Can you work these out from the model? Positions are in its coordinate system, mm. A direction names the side the tool comes from. Give positions to 0.01 mm unless a question says otherwise; leave off trailing zeros. Write each loop counter-clockwise with the first axis right and the second up, starting at its lowest first coordinate (ties: lowest second). Pieces come first, ordered by that corner, then holes. Notation, with made-up numbers: (8.25, 57.25) -> (27.25, 57.25) arc R28 ccw to (27.25, 91.25) -> close; hole circle Ø6 at (-14, 82). An arc over 180 degrees is marked (long way). Answer as CSV lines item,"result". Start each with the question number.
1. I need wall thicknesses on line 1 (X direction, y = -3.5, z = 160); line 2 (Z direction, x = -81.5, y = 8.5); line 3 (X direction, y = 13, z = 170). Which ranges of each line are inside material? Lowest first, please. Write a range as [from, to].
2. If we section it at B-B on y = -6.5: Write out the boundary of the cut face in (x, z).
3. I'm going to push flat-ended pins straight in: P1, Ø5, axis at y = 20, z = 117, coming from the -X side; P2, Ø5, axis at y = 20.5, z = 169.5, coming from the +X side; P3, Ø9.5, axis at y = 10, z = 165.5, coming from the -X side; P4, Ø4, axis at x = -64.5, z = 109, coming from the -Y side. Where does each tip first touch, or does it pass through?
4. If we section it at A-A on z = 135: Write out the boundary of the cut face in (x, y), plus the area to 3 significant figures.
5. If we mould it in two halves opening along X, with no side actions, what happens to faces 1 (the face through (-106.579, 10, 169)), 2 (the face through (-67.574, -4.93, 159.78)), 3 (the face through (-29.5, -4.9, 107.5)), 4 (the face through (-92, -3, 91))? For each: pulls with the +X half, pulls with the -X half, needs draft (parallel to the pull), parting line crosses it, or undercut.
6. If we section it at C-C on x = -109.5: Write out the boundary of the cut face in (y, z), plus the area to 3 significant figures.
7. On a 3-axis mill with a long thin cutter (end or side, diameter ignored), from which of +Z, -Z, +X, -X, +Y, -Y can I reach the whole of each face in a straight line? I mean faces 5 (the face through (-106.579, 10, 100)), 6 (the face through (-93.579, 15, 99)), 7 (the face through (-90.579, 15, 150)). Say none if no direction works.
Autodesk Fusion 360 part; units mm, degrees
sketch "Sketch1" plane through (0, 0, 0) normal (0, 1, 0) x (1, 0, 0)
  line L0 (-93.5789, -91) -> (-48.797, -91)
  line L1 (-48.797, -91) -> (-48.797, -179)
  line L2 (-48.797, -179) -> (-93.5789, -179)
  line L3 (-93.5789, -179) -> (-93.5789, -91)
  line L4 (-48.797, -179) -> (2.6553, -135)
  line L5 (2.6553, -135) -> (-48.797, -91)
  line L6 (-93.5789, -91) -> (-148.2679, -91)
  line L7 (-148.2679, -91) -> (-148.2679, -179)
  line L8 (-148.2679, -179) -> (-93.5789, -179)
  line L9 (2.6553, -135) -> (-148.2679, -135)
  line L10 (-90.5789, -91) -> (-90.5789, -179)
  line L11 (-26.5789, -110) -> (-26.5789, -160)
  line L12 (-26.5789, -130) -> (-90.5789, -130)
  line L13 (-26.5789, -140) -> (-90.5789, -140)
  line L14 (-26.5789, -110) -> (-90.5789, -110)
  line L15 (-26.5789, -160) -> (-90.5789, -160)
  line L16 (-62.5789, -91) -> (-62.5789, -179)
  circle A0 centre (-62.5789, -110) radius 5
  circle A1 centre (-62.5789, -160) radius 5
  line L17 (-106.5789, -91) -> (-106.5789, -179)
  line L18 (-112.5789, -91) -> (-112.5789, -179)
  line L19 (-86.5789, -140) -> (-86.5789, -130)
  circle A2 centre (-112.5789, -135) radius 9.5
  circle A3 centre (-112.5789, -135) radius 19
  line L20 (-26.5789, -135) -> (-14.2304, -120.56)
  line L21 (-26.5789, -135) -> (-14.2304, -149.44)
  circle A4 centre (-26.5789, -135) radius 19
  line L22 (-90.5789, -160) -> (-93.5789, -160)
  line L23 (-90.5789, -130) -> (-93.5789, -130)
  line L24 (-90.5789, -110) -> (-93.5789, -110)
  line L25 (-90.5789, -140) -> (-93.5789, -140)
  dimension "d1" = 3
  dimension "d2" = 5
  dimension "d3" = 10
  dimension "d4" = 50
  dimension "d7" = 88
  dimension "d8" = 67
  dimension "d10" = 31
  dimension "d11" = 36
  dimension "d12" = 10
  dimension "d13" = 10
  dimension "d16" = 13
  dimension "d17" = 19
  dimension "d18" = 20
  dimension "d19" = 19
  dimension "d20" = 38
  dimension "d22" = 19
  dimension "d23" = 19
  dimension "d24" = 13.782
extrude "Extrude1" add sketch "Sketch1" against normal blind 10 contours L0 L3 L10 L24 | L3 L6 L17 A3 | L0 L10 L14 L16 A0 | L3 L10 L23 L24 | L0 L1 L14 L16 A0 | L10 L12 L14 L16 A0 | L3 L9 L10 L23 | L9 L17 A2 A3 | L17 L18 A2 A3 | L1 L5 L14 | L9 L10 L12 L19 | L3 L9 L10 L25 | L9 L17 A2 A3 | L3 L8 L17 A3 | L9 L18 A2 A3 | L1 L11 L12 L14 A4 | L1 L12 L14 L16 A0 | L5 L11 A4 | L9 L10 L13 L19 | L9 L12 L16 L19 | L3 L10 L22 L25 | L17 L18 A2 A3 | L9 L18 A2 A3 | L1 L9 L12 A4 | L1 L9 L12 L16 | L9 L20 A4 | L11 L20 A4 | L11 L12 A4 | L9 L13 L16 L19 | L10 L13 L15 L16 A1 | L2 L3 L10 L22 | L1 L9 L13 A4 | L1 L9 L13 L16 | L9 L11 L12 A4 | L9 L11 L13 A4 | L11 L21 A4 | L9 L21 A4 | L2 L10 L15 L16 A1 | L1 L11 L13 L15 A4 | L1 L13 L15 L16 A1 | L4 L11 A4 | L11 L13 A4 | L1 L4 L15 | L1 L2 L15 L16 A1 makes body 1
extrude "Extrude2" add sketch "Sketch1" along normal blind 30 contours L3 L6 L17 A3 | L3 L10 L23 L24 | L3 L9 L10 L23 | L9 L17 A2 A3 | L17 L18 A2 A3 | L9 L10 L12 L19 | L3 L9 L10 L25 | L9 L17 A2 A3 | L3 L8 L17 A3 | L9 L18 A2 A3 | L9 L10 L13 L19 | L3 L10 L22 L25 | L17 L18 A2 A3 | L9 L18 A2 A3 bodies 1
extrude "Extrude3" add sketch "Sketch1" along normal blind 30 separate body contours L9 L12 L16 L19 | L1 L9 L12 A4 | L1 L9 L12 L16 | L9 L13 L16 L19 | L1 L9 L13 A4 | L1 L9 L13 L16 | L9 L11 L12 A4 | L9 L11 L13 A4 makes body 2
draft "Draft1" angle -26.5 neutral plane through (-86.5789, 0, 135) pull (-1, 0, 0) 1 faces at (-46.5789, 30, 133.3333) on bodies 2
combine "Combine1" operation add target body 2 tool bodies 1
fillet "Fillet1" radius 13 1 edges at (-48.797, -5, 179) on bodies 2
fillet "Fillet2" radius 13 1 edges at (-48.797, -5, 91) on bodies 2
fillet "Fillet3" radius 3 1 edges at (-93.5789, 15, 160) on bodies 2
fillet "Fillet4" radius 3 1 edges at (-93.5789, 15, 110) on bodies 2
fillet "Fillet5" radius 6 1 edges at (-106.5789, 10, 153.0278) on bodies 2
fillet "Fillet6" radius 6 1 edges at (-106.5789, 10, 116.9722) on bodies 2
Computed values:
1,line 1,"x = [-106.58, -67.58], [-57.58, -26.58]"
1,line 2,"z = [130, 140]"
1,line 3,"x = [-106.58, -93.58]"
2,outline,"(-112.58, 116) arc R6 cw to (-106.58, 110) -> (-106.58, 91) -> (-53.6, 91) arc R13 ccw to (-45.15, 94.12) -> (-14.23, 120.56) arc R19 ccw to (-14.23, 149.44) -> (-45.15, 175.88) arc R13 ccw to (-53.6, 179) -> (-106.58, 179) -> (-106.58, 160) arc R6 cw to (-112.58, 154) arc R19 ccw to start; hole circle Ø19 at (-112.58, 135); hole circle Ø10 at (-62.58, 110); hole circle Ø10 at (-62.58, 160)"
3,P1,"stops at x = -123.57"
3,P2,"stops at x = -93.58"
3,P3,"stops at x = -106.58"
3,P4,"passes through"
4,outline,"(-131.58, -10) -> (-122.08, -10) -> (-122.08, 30) -> (-131.58, 30) -> close; (-103.08, -10) -> (-7.58, -10) -> (-7.58, 0) -> (-26.58, 0) -> (-26.58, 0.09) -> (-86.58, 30) -> (-103.08, 30) -> close"
4,area,"2,730 mm2"
5,face 1,"pulls with the -X half"
5,face 2,"undercut"
5,face 3,"pulls with the +X half"
5,face 4,"needs draft"
6,outline,"(-10, 115.15) -> (30, 115.15) -> (30, 126.01) -> (-10, 126.01) -> close; (-10, 143.99) -> (30, 143.99) -> (30, 154.85) -> (-10, 154.85) -> close"
6,area,"869 mm2"
7,face 5,"-Z, -X, +Y, -Y"
7,face 6,"-Z, +X, +Y"
7,face 7,"+Z, +X, +Y"
